Input: part model. Units: mm. Frame: model coordinates. Coordinates: 2 decimals unless noted, no trailing zeros. Loops run counter-clockwise (first coordinate to the right, second up) from the corner with the lowest first, then second, coordinate; pieces in that order, holes last.
(1) Line query: L1, parallel to Z at x = -1, y = 1.1; L2, parallel to X at y = 1.75, z = -1; L3, parallel to Z at x = 2.75, y = 1.75. Output: solid intervals per line, ascending.
(2) Section B-B, the plane y = 0.5. Return loops of the section in (x, z).
(3) Section A-A, the plane y = 1.5. Return loops of the section in (x, z), then the cut area to 3 significant figures.
(4) Contact query for flat-ended pins moving along their axis: P1, Ø1, axis at y = 2, z = 4, coming from the +X side; P2, Ø1.5, axis at x = 4, z = -3, coming from the +Y side. Output: stop coordinate, or through.
(5) Mould query, pull axis X, two halves, no side actions, for faces 1 (the face through (-3.07, 1.23, -4.01)), 2 (the face through (6.12, 1.23, 3.6)), 3 (the face through (-2, 0, -5)). Classes: released by +X, released by -X, zero draft, split by the parting line, or undercut.
```python
from build123d import *

# Parameters (mm, degrees)
SKIZZE1_R                       = 5.05
AUFSATZ_LINEAR_AUSTRAGEN1_DEPTH = 2.5


with BuildPart() as part:
    # Skizze1 → Aufsatz-Linear austragen1 (new body)
    with BuildSketch(Plane(origin=(0, 0, 0), x_dir=(1, 0, 0), z_dir=(0, 1, 0))):
        Polygon((8.198373822, 0), (4.099186911, 7.1), (-4.099186911, 7.1), (-8.198373822, 0), (-4.099186911, -7.1), (4.099186911, -7.1), align=None)
        with Locations(Location((0, 0, 0), (0, 0, 270))):
            Circle(SKIZZE1_R, mode=Mode.SUBTRACT)
    extrude(amount=AUFSATZ_LINEAR_AUSTRAGEN1_DEPTH)

    # Skizze4 → Schnitt-Rotation1 (revolve, cut)
    with BuildSketch(Plane(origin=(0, 0, 0), x_dir=(0.49999999999999506, 0, -0.8660254037844415), z_dir=(0.8660254037844415, 0, 0.49999999999999506))):
        Polygon((-8.198373822, 0.75), (-7.1, 0), (-8.198373822, 0), align=None)
    schnitt_rotation1 = revolve(axis=Axis((0, 0, 0), (0, 1, 0)), mode=Mode.SUBTRACT)

    # Spiegeln1: Schnitt-Rotation1 across plane
    add(schnitt_rotation1.mirror(Plane.ZX.offset(1.25)), mode=Mode.SUBTRACT)


solid = part.part
```
Report:
1. L1: z = -7.1 to -4.95, 4.95 to 7.1
1. L2: x = -7.62 to -4.95, 4.95 to 7.62
1. L3: z = -7.1 to -4.24, 4.24 to 7.1
2. outline: (-7.8, -0.69) - (-4.5, -6.41) arc R7.83 ccw to (-3.31, -7.1) - (3.31, -7.1) arc R7.83 ccw to (4.5, -6.41) - (7.8, -0.69) arc R7.83 ccw to (7.8, 0.69) - (4.5, 6.41) arc R7.83 ccw to (3.31, 7.1) - (-3.31, 7.1) arc R7.83 ccw to (-4.5, 6.41) - (-7.8, 0.69) arc R7.83 ccw to start; hole circle Ø10.1 at (0, 0)
3. outline: (-8.2, 0) - (-4.1, -7.1) - (4.1, -7.1) - (8.2, 0) - (4.1, 7.1) - (-4.1, 7.1) - close; hole circle Ø10.1 at (0, 0)
3. area: 94.5 mm2
4. P1: stops at x = 6.18
4. P2: stops at y = 2.5
5. face 1: undercut
5. face 2: released by +X
5. face 3: zero draft
